CAD build for the part. Positions are in the model's coordinates, mm. A direction names the side the tool comes from. Give positions to 0.01 mm unless a question says otherwise; leave off trailing zeros. Put each result on its own line as item: value. Start each with the question number.
1) Pin check, flat tips, straight feed: pin 1 (4 mm diameter, centred on x = -4.5, z = -11, fed in from -Y); pin 2 (1 mm diameter, centred on x = -8, z = -14, fed in from +Y). Stop position of each tip, or through.
2) Drill centre lines: line 1 (X direction, y = 0.35, z = -10.25); line 2 (X direction, y = 1.3, z = -10.25); line 3 (Z direction, x = 0, y = 1.5). Where is each one in solid material? Low to high. Write a range as [from, to].
3) Two-plate mould, pull along X, no slides. Class faces 1 (the face through (0, 1.27, -14.5)), 2 (the face through (10.533, 0.644, -11.267)), 3 (the face through (0.1, 1.8, -12.7)): released by +X, released by -X, zero draft, split by the parting line, or undercut.
4) Tool access for faces 4 (the face through (9.5, 1, -9.5)), 5 (the face through (-0.16, 1.65, -14.16)): list every direction of +Z, -Z, +X, -X, +Y, -Y with a clear straight run to the whole face (end or side of a thin tool).
```python
from build123d import *

# Parameters (mm, degrees)
BOSS_EXTRUDE1_DEPTH = 2.032
CUT_EXTRUDE1_START  = -0.762
CUT_EXTRUDE1_DEPTH  = 0.762
FILLET2_R           = 1.524
FILLET1_R           = 1.524


with BuildPart() as part:
    # Sketch1 → Boss-Extrude1 (new body)
    with BuildSketch(Plane(origin=(0, 0, 0), x_dir=(1, 0, 0), z_dir=(0, 1, 0))):
        with BuildLine():
            Line((-8.980256121, 8.980256121), (-11.225320151, 11.225320151))
            ThreePointArc((-11.225320151, 11.225320151), (0, 15.875), (11.225320151, 11.225320151))
            Line((11.225320151, 11.225320151), (8.980256121, 8.980256121))
            ThreePointArc((8.980256121, 8.980256121), (0, 12.7), (-8.980256121, 8.980256121))
        make_face()
    extrude(amount=BOSS_EXTRUDE1_DEPTH)

    # Sketch2 → Cut-Extrude1 (cut)
    with BuildSketch(Plane(origin=(0, 2.032, 0), x_dir=(1, 0, 0), z_dir=(0, 1, 0)).offset(CUT_EXTRUDE1_START)):
        with BuildLine():
            Line((10.012985575, 10.012985575), (11.225320151, 11.225320151))
            ThreePointArc((11.225320151, 11.225320151), (0, 15.875), (-11.225320151, 11.225320151))
            Line((-11.225320151, 11.225320151), (-10.012985575, 10.012985575))
            ThreePointArc((-10.012985575, 10.012985575), (0, 14.1605), (10.012985575, 10.012985575))
        make_face()
    extrude(amount=CUT_EXTRUDE1_DEPTH, mode=Mode.SUBTRACT)

    # Fillet2
    fillet2_edges = [part.edges().sort_by_distance(p)[0] for p in [
        (0, 0, -12.7),
    ]]
    fillet(fillet2_edges, radius=FILLET2_R)

    # Fillet1
    fillet1_edges = [part.edges().sort_by_distance(p)[0] for p in [
        (-11.225320151, 0.635, -11.225320151),
        (11.225320151, 0.635, -11.225320151),
    ]]
    fillet(fillet1_edges, radius=FILLET1_R)


solid = part.part
```
Solution:
1. pin 1: y = 0.04
1. pin 2: y = 1.27
2. line 1: [-10.23, -8.4], [8.4, 10.23]
2. line 2: [-9.77, -7.53], [7.53, 9.77]
2. line 3: [-14.16, -12.7]
3. face 1: zero draft
3. face 2: released by +X
3. face 3: undercut
4. face 4: +Z, +X, +Y, -Y
4. face 5: -Z, +Y
